Design review of the part built by this model. Coordinates are the model's own, in mm. A direction names the side the tool comes from. Coordinates: 2 decimals unless noted, no trailing zeros. Loops run counter-clockwise (first coordinate to the right, second up) from the corner with the lowest first, then second, coordinate; pieces in that order, holes last. Notation, with made-up numbers: M 62.5,22 L 106.5,22 A24 ccw 106.5,59 Z; hole C 15.5,-17.5 d7. An arc over 180 degrees is marked long. Put each result on its own line as item: value. Start each with the question number.
(1) For faces 1 (the flat face through (9, 0, 12)), 2 (the flat face through (9, 0, -12)), 3 (the flat face through (-1, -1.5, 0)), list the 3-axis set-ups (+Z, -Z, +X, -X, +Y, -Y) from which the entire face can be reached by the end or side of a thin tool; tool diameter is ignored.
(2) For probe 1 along Z at (x, y) = (-12.5, -0.5); probe 2 along X at (y, z) = (-0.65, -2.25); probe 3 along X at (y, z) = (-1, -6.5), list the stretches that pass through material, from the lowest coordinate up. Write a range as [from, to].
(3) Take a section at A-A, the plane x = 12.5. Give the boundary of the cut face in (y, z) (3 decimals).
(4) Clearance check with flat-ended pins moving along their axes: pin 1 (1.5 mm diameter, centred on y = 0.5, z = -13.5, fed in from -X); pin 2 (0.9 mm diameter, centred on x = -46.5, y = 0, fed in from -Z); pin 3 (1.5 mm diameter, centred on y = 0.5, z = 13, fed in from +X). State where each tip first meets the part, or that it passes through.
(5) The part is to be moulded in two halves that separate along X. For faces 4 (the flat face through (-55, 0, -4.5)), 5 (the flat face through (-9, 0, 12)), 6 (the flat face through (54, 0, 10)), say which applies: +X half, -X half, draft (parallel to the pull), parting line (faces both ways), or undercut.
(6) Take a section at D-D, the plane z = 8. Give the boundary of the cut face in (x, y), then the cut area to 3 significant figures.
(7) Take a section at B-B, the plane y = -0.4. Count the separate pieces of the cut face and the enclosed holes in it, then the cut area to 3 significant figures.
(8) Take a section at C-C, the plane x = -46.5. Give the boundary of the cut face in (y, z), then the cut area to 3 significant figures.
```python
from build123d import *

# Parameters (mm, degrees)
BOSS_EXTRUDE1_DEPTH            = 1.5
M5_CLEARANCE_HOLE1_D           = 5.5
M5_CLEARANCE_HOLE1_CSINK_D     = 5.55
M5_CLEARANCE_HOLE1_CSINK_ANGLE = 90


with BuildPart() as part:
    # Sketch1 → Boss-Extrude1 (new, symmetric)
    with BuildSketch(Plane(origin=(0, 0, 0), x_dir=(1, 0, 0), z_dir=(0, 1, 0))):
        Polygon((54, 15), (49.5, 15), (49.5, 12), (40.5, 12), (40.5, 15), (31.5, 15), (31.5, 12), (22.5, 12), (22.5, 15), (13.5, 15), (13.5, 12), (4.5, 12), (4.5, 15), (-4.5, 15), (-4.5, 12), (-13.5, 12), (-13.5, 15), (-22.5, 15), (-22.5, 12), (-31.5, 12), (-31.5, 15), (-40.5, 15), (-40.5, 12), (-49.5, 12), (-49.5, 15), (-54, 15), (-54, 12), (-54, 4.5), (-57, 4.5), (-57, -4.5), (-54, -4.5), (-54, -12), (-54, -15), (-49.5, -15), (-49.5, -12), (-40.5, -12), (-40.5, -15), (-31.5, -15), (-31.5, -12), (-22.5, -12), (-22.5, -15), (-13.5, -15), (-13.5, -12), (-4.5, -12), (-4.5, -15), (4.5, -15), (4.5, -12), (13.5, -12), (13.5, -15), (22.5, -15), (22.5, -12), (31.5, -12), (31.5, -15), (40.5, -15), (40.5, -12), (49.5, -12), (49.5, -15), (54, -15), (54, -12), (54, -4.5), (57, -4.5), (57, 4.5), (54, 4.5), (54, 12), align=None)
    extrude(amount=BOSS_EXTRUDE1_DEPTH, both=True)

    # M5 Clearance Hole1 (through all)
    with Locations(Plane(origin=(0, 1.5, 0), x_dir=(1, 0, 0), z_dir=(0, 1, 0))):
        with Locations((-12.5, 4.5), (12.5, 4.5)):
            CounterSinkHole(M5_CLEARANCE_HOLE1_D / 2, M5_CLEARANCE_HOLE1_CSINK_D / 2, counter_sink_angle=M5_CLEARANCE_HOLE1_CSINK_ANGLE)


solid = part.part
```
Computed values:
1. face 1: +Z, +Y, -Y
1. face 2: -Z, +Y, -Y
1. face 3: +Z, -Z, +X, -X, -Y
2. probe 1: z = [-12, -7.25], [-1.75, 12]
2. probe 2: x = [-57, -14.08], [-10.92, 10.92], [14.08, 57]
2. probe 3: x = [-54, -14.39], [-10.61, 10.61], [14.39, 54]
3. outline: M -1.5,-12 L 1.5,-12 L 1.5,-7.275 L 1.475,-7.25 L -1.5,-7.25 Z; M -1.5,-1.75 L 1.475,-1.75 L 1.5,-1.725 L 1.5,12 L -1.5,12 Z
4. pin 1: stops at x = -54
4. pin 2: stops at z = -12
4. pin 3: stops at x = 54
5. face 4: draft
5. face 5: undercut
5. face 6: +X half
6. outline: M -54,-1.5 L 54,-1.5 L 54,1.5 L -54,1.5 Z
6. area: 324 mm^2
7. separate pieces: 1
7. enclosed holes: 2
7. area: 2,920 mm^2
8. outline: M -1.5,-12 L 1.5,-12 L 1.5,12 L -1.5,12 Z
8. area: 72.0 mm^2
